from build123d import *

# Parameters (mm, degrees)
F0_W     = 3.175
F0_H     = 3.175
F1_DEPTH = 6.35
F2_W     = 3.175
F2_H     = 4.0921564981
F2_H_2   = 0.1173117965
F2_H_3   = 3.9748447016
F2_W_2   = 4.0921564981
F2_H_4   = 3.175
F3_DEPTH = 25.4


with BuildPart() as f1:
    # F0 (on Top) → F1 (new body)
    with BuildSketch(Plane.XY):
        with Locations((-11.1125, 11.1125)):
            Rectangle(F0_W, F0_H)
        with Locations((11.1125, 11.1125)):
            Rectangle(F0_W, F0_H)
        with Locations((11.1125, -11.1125)):
            Rectangle(F0_W, F0_H)
        with Locations((-11.1125, -11.1125)):
            Rectangle(F0_W, F0_H)
        Polygon((6.35, 9.525), (9.525, 12.7), (-9.525, 12.7), (-6.35, 9.525), align=None)
        Polygon((-9.525, -12.7), (9.525, -12.7), (6.35, -9.525), (-6.35, -9.525), align=None)
        Polygon((12.7, -9.525), (12.7, 9.525), (9.525, 6.35), (9.525, -6.35), align=None)
        Polygon((-9.525, 6.35), (-12.7, 9.525), (-12.7, -9.525), (-9.525, -6.35), align=None)
        Polygon((9.525, 9.525), (9.525, 12.7), (6.35, 9.525), align=None)
        Polygon((-6.35, 9.525), (-9.525, 12.7), (-9.525, 9.525), align=None)
        Polygon((9.525, -12.7), (9.525, -9.525), (6.35, -9.525), align=None)
        Polygon((-9.525, -9.525), (-9.525, -12.7), (-6.35, -9.525), align=None)
        Polygon((9.525, 6.35), (12.7, 9.525), (9.525, 9.525), align=None)
        Polygon((9.525, -9.525), (12.7, -9.525), (9.525, -6.35), align=None)
        Polygon((-9.525, 6.35), (-9.525, 9.525), (-12.7, 9.525), align=None)
        Polygon((-9.525, -6.35), (-12.7, -9.525), (-9.525, -9.525), align=None)
        Polygon((9.525, 6.35), (9.525, 9.525), (6.35, 9.525), (0, 3.175), (3.175, 0), align=None)
        Polygon((-6.35, 9.525), (-9.525, 9.525), (-9.525, 6.35), (-3.175, 0), (0, 3.175), align=None)
        Polygon((6.35, -9.525), (9.525, -9.525), (9.525, -6.35), (3.175, 0), (0, -3.175), align=None)
        Polygon((3.175, 0), (0, 3.175), (-3.175, 0), (0, -3.175), align=None)
        Polygon((0, -3.175), (-3.175, 0), (-9.525, -6.35), (-9.525, -9.525), (-6.35, -9.525), align=None)
    extrude(amount=F1_DEPTH)

    # F2 (on face) → F3 (cut)
    with BuildSketch(Plane(origin=(0, 0, 0), x_dir=(1, 0, 0), z_dir=(0, 0, -1))):
        with Locations((11.1125, 0.0586558983)):
            Rectangle(F2_W, F2_H)
        with Locations((-11.1125, 2.0460782491)):
            Rectangle(F2_W, F2_H_2)
        with Locations((-11.1125, 0)):
            Rectangle(F2_W, F2_H_3)
        with Locations((-11.1125, -2.0460782491)):
            Rectangle(F2_W, F2_H_2)
        with Locations((-0.0586558983, 11.1125)):
            Rectangle(F2_W_2, F2_H_4)
        with Locations((0.0586558983, -11.1125)):
            Rectangle(F2_W_2, F2_H_4)
    extrude(amount=-F3_DEPTH, mode=Mode.SUBTRACT)


solid = f1.part
Build history of the part. All positions in model axes, mm. A direction names the side the tool comes from. Give positions to 0.01 mm unless a question says otherwise; leave off trailing zeros. Order: outer loops, then holes, each group sorted by start corner. A loop starts at its lowest first (then second) coordinate and runs counter-clockwise, first axis right, second up. Notation, with made-up numbers: M -5,-36 L 4,-36 A25 ccw 4,-4 Z; hole C 40,24 d5. An arc over 180 degrees is marked long. Put each result on its own line as item: value.
Item 1: Two-plate mould, pull along X, no slides. Class faces 4 (the flat face through (7, 12.7, 3)), 5 (the flat face through (-6.306, -3.131, 3.131)), 6 (the flat face through (-12.7, 7, 3)): +X half, -X half, draft (parallel to the pull), parting line (faces both ways), or undercut.
From the geometry:
face 4: draft
face 5: undercut
face 6: -X half
Item 2: Slice it at A-A, the plane x = 10. Write the cut outline in (y, z), plus the area to 3 significant figures.
From the geometry:
outline: M -12.7,0 L -2.1,0 L -2.1,6.35 L -12.7,6.35 Z; M 1.99,0 L 12.7,0 L 12.7,6.35 L 1.99,6.35 Z
area: 135 mm2
Item 3: 3-axis set-ups, long thin cutter, end or side, ignore diameter. For faces 1 (the flat face through (-3.131, 6.306, 3.131)), 2 (the flat face through (-2.105, -11, 3)), 3 (the flat face through (11, -2.105, 3)): which of +Z, -Z, +X, -X, +Y, -Y reach the whole face in a straight line?
From the geometry:
face 1: +Z, -Z
face 2: +Z, -Z, -Y
face 3: +Z, -Z, +X
Item 4: Probe line 1 (Y direction, x = 4.75, z = 0.5) (3 decimals); line 2 (Y direction, x = -6, z = 3.25) (3 decimals); line 3 (X direction, y = 9.75, z = 5.5). List the from-to ranges inside material, lowest first. Write a range as [from, to].
From the geometry:
line 1: y = [-12.7, -9.525], [-7.925, -1.575], [1.575, 7.925], [9.525, 12.7]
line 2: y = [-12.7, -9.525], [-9.175, -2.825], [2.825, 9.175], [9.525, 12.7]
line 3: x = [-12.7, -1.99], [2.1, 12.7]
Item 5: Slice it at C-C, the plane y = 2.5. Write the cut outline in (x, z) (3 decimals), plus the area to 3 significant figures.
From the geometry:
outline: M -12.7,0 L -9.525,0 L -9.525,6.35 L -12.7,6.35 Z; M -5.675,0 L 5.675,0 L 5.675,6.35 L -5.675,6.35 Z; M 9.525,0 L 12.7,0 L 12.7,6.35 L 9.525,6.35 Z
area: 112 mm2
Item 6: Flat gauge pin, fed straight in: pin 1 Ø1 at (y, z) = (0.5, 5.5) entering from -X (3 decimals). Where does the tip first touch, or does it go through?
From the geometry:
pin 1: stops at x = -4.175
